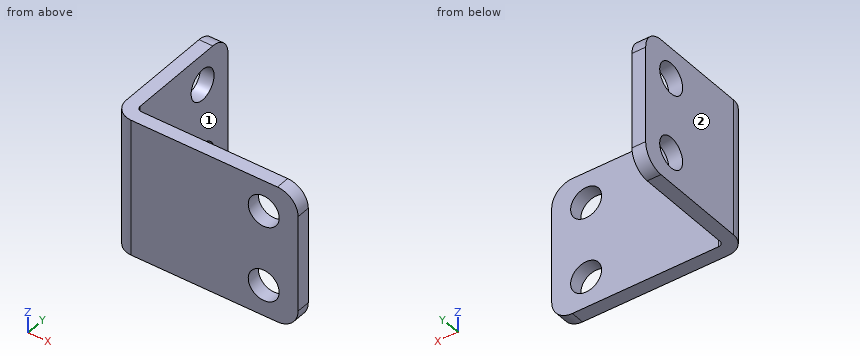
```python
from build123d import *

# Parameters (mm, degrees)
SM_BASE_FLANGE_1_DEPTH = 10
SKETCH_3_R             = 2.25
CUT_EXTRUDE_1_DEPTH    = 34.541019662
SKETCH_4_R             = 2.25
CUT_EXTRUDE_2_DEPTH    = 34.955853693
FILLET_1_R             = 3


# Sheet-metal steps are written as plain solids
with BuildPart() as part:
    # Sketch 1 → 基体-法兰1 (new, symmetric)
    with BuildSketch(Plane.XY):
        with BuildLine():
            Line((0, 20), (0, 2.7366))
            ThreePointArc((0, 2.7366), (0.801531583, 0.801531583), (2.7366, 0))
            Line((2.7366, 0), (27, 0))
            Line((27, 0), (27, 2))
            Line((27, 2), (2.7366, 2))
            ThreePointArc((2.7366, 2), (2.215745145, 2.215745145), (2, 2.7366))
            Line((2, 2.7366), (2, 20))
            Line((2, 20), (0, 20))
        make_face()
    extrude(amount=SM_BASE_FLANGE_1_DEPTH, both=True)

    # 草图3 → 切除-拉伸1 (cut, through all)
    with BuildSketch(Plane(origin=(2, 0, 0), x_dir=(0, 0, -1), z_dir=(1, 0, 0))):
        with Locations(Location((-5.5, 15, 0), (0, 0, 90))):
            Circle(SKETCH_3_R)
        with Locations(Location((5.5, 15, 0), (0, 0, 270))):
            Circle(SKETCH_3_R)
    extrude(amount=-CUT_EXTRUDE_1_DEPTH, mode=Mode.SUBTRACT)

    # 草图4 → 切除-拉伸2 (cut, through all)
    with BuildSketch(Plane(origin=(0, 2, 0), x_dir=(1, 0, 0), z_dir=(0, 1, 0))):
        with Locations(Location((22, 5.5, 0), (0, 0, 270))):
            Circle(SKETCH_4_R)
        with Locations(Location((22, -5.5, 0), (0, 0, 90))):
            Circle(SKETCH_4_R)
    extrude(amount=-CUT_EXTRUDE_2_DEPTH, mode=Mode.SUBTRACT)

    # 圆角1
    fillet_1_edges = [part.edges().sort_by_distance(p)[0] for p in [
        (1, 20, 10),
        (27, 1, 10),
        (1, 20, -10),
        (27, 1, -10),
    ]]
    fillet(fillet_1_edges, radius=FILLET_1_R)


solid = part.part
```
Here's how the part is built. I have some questions about the finished solid (model axes, mm). Face numbers are marked on the shaded views. A direction names the side the tool comes from. Coordinates: 2 decimals unless noted, no trailing zeros. Loops run counter-clockwise (first coordinate to the right, second up) from the corner with the lowest first, then second, coordinate; pieces in that order, holes last. Notation, with made-up numbers: (-6.5, 83) -> (18.5, 83) arc R27 cw to (18.5, 122) -> close; hole circle Ø8 at (65, -37.75). An arc over 180 degrees is marked (long way). Return JSON: item names as keys, results as strings.
1) For the marked faces 1 and 2, which set-ups out of +Z, -Z, +X, -X, +Y, -Y let a thin tool reach every point of the face, with its end or its side?
Results below:
{"face 1": "+Z, -Z, +X, +Y", "face 2": "+Z, -Z, -X, +Y, -Y"}
2) I need wall thicknesses on line 1 (Z direction, x = 1.55, y = 15); line 2 (X direction, y = 19.25, z = -6.5). Which ranges of each line are inside material? Lowest first, please. Write a range as from..to.
Results below:
{"line 1": "-10..-7.75, -3.25..3.25, 7.75..10", "line 2": "0..2"}
3) If we section it at C-C, the plane z = 5.5: Write out the boundary of the cut face in (x, y), then the cut area to 3 significant figures.
Results below:
{"outline": "(0, 2.74) arc R2.74 ccw to (2.74, 0) -> (19.75, 0) -> (19.75, 2) -> (2.74, 2) arc R0.74 cw to (2, 2.74) -> (2, 12.75) -> (0, 12.75) -> close; (0, 17.25) -> (2, 17.25) -> (2, 20) -> (0, 20) -> close; (24.25, 0) -> (27, 0) -> (27, 2) -> (24.25, 2) -> close", "area": "70.5 mm²"}
4) Will these pins go through, and if not, where does the flat tip stop? pin 1 (3.5 mm diameter, centred on y = 15, z = -5.5, fed in from +X); pin 2 (1 mm diameter, centred on x = 21.5, z = 1, fed in from +Y); pin 3 (12 mm diameter, centred on y = 18, z = -6, fed in from +X); pin 4 (6 mm diameter, centred on x = 22, z = -5.5, fed in from -Y).
Results below:
{"pin 1": "through", "pin 2": "y = 2", "pin 3": "x = 2", "pin 4": "y = 0"}
5) If we section it at D-D, the plane x = 15.5: Write out the boundary of the cut face in (y, z).
Results below:
{"outline": "(0, -10) -> (2, -10) -> (2, 10) -> (0, 10) -> close"}
6) If we section it at A-A, the plane x = 22: Write out the boundary of the cut face in (y, z).
Results below:
{"outline": "(0, -10) -> (2, -10) -> (2, -7.75) -> (0, -7.75) -> close; (0, -3.25) -> (2, -3.25) -> (2, 3.25) -> (0, 3.25) -> close; (0, 7.75) -> (2, 7.75) -> (2, 10) -> (0, 10) -> close"}
